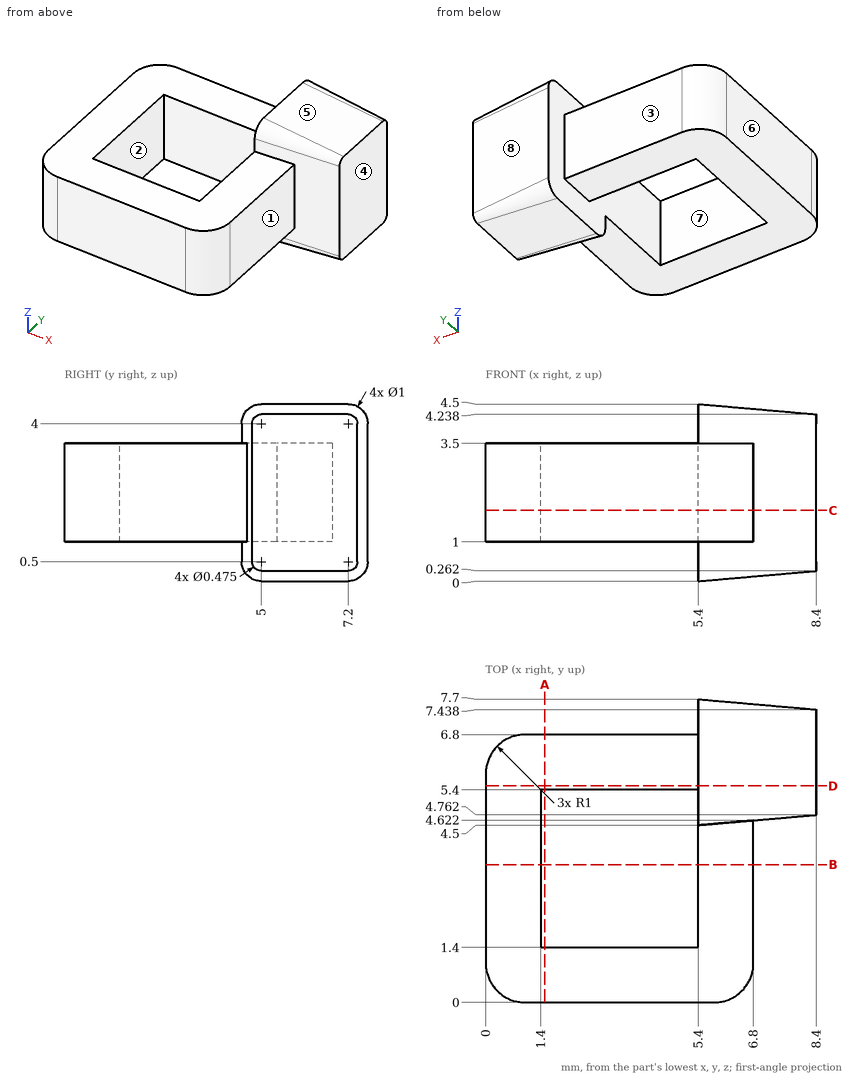
Could you check a few things on this drawing? It's one solid part, dimensions in mm from its lowest x, y, z. A direction names the side the tool comes from. Give positions to 0.01 mm unless a question says otherwise; leave off trailing zeros. Loops run counter-clockwise (first coordinate to the right, second up) from the corner with the lowest first, then second, coordinate; pieces in that order, holes last. Notation, with made-up numbers: M 75.25,-23.75 L 117.25,-23.75 A12 ccw 117.25,-9.75 Z; hole C 85.5,-14 d8. An arc over 180 degrees is marked long. Answer as a JSON object with one key per item and string values.
Q1. Suppose I cut it at D-D, the plane y = 5.5. List the corners of the cut face in (x, z) for me, plus the area to 3 significant figures.
Values found:
{"outline": "M 0,1 L 5.4,1 L 5.4,0 L 8.4,0.26 L 8.4,4.24 L 5.4,4.5 L 5.4,3.5 L 0,3.5 Z", "area": "26.2 mm²"}
Q2. Suppose I cut it at A-A, the plane x = 1.5. List the corners of the cut face in (y, z) for me.
Values found:
{"outline": "M 0,1 L 1.4,1 L 1.4,3.5 L 0,3.5 Z; M 5.4,1 L 6.8,1 L 6.8,3.5 L 5.4,3.5 Z"}
Q3. For the marked faces 1, 2, 3, 4 and 5, which set-ups out of +Z, -Z, +X, -X, +Y, -Y let a thin tool reach every point of the face, with its end or its side?
Values found:
{"face 1": "+Z, -Z, +X, -Y", "face 2": "+Z, -Z", "face 3": "+Z, -Z, -X, +Y", "face 4": "+Z, -Z, +X, +Y, -Y", "face 5": "+Z, +X, +Y, -Y"}
Q4. If I drill on probe 1 along X at (y, z) = (5.25, 1.8); probe 2 along Y at (x, z) = (3.25, 2), over which ranges is the centre line in solid material (lowest first)? Write a range as [from, to].
Values found:
{"probe 1": "x = [0, 1.4], [5.4, 8.4]", "probe 2": "y = [0, 1.4], [5.4, 6.8]"}
Q5. For P1, Ø2, axis at y = 2.5, z = 2.5, coming from the +X side; P2, Ø1, axis at x = 5, y = 3.5, coming from the +Z side; P3, Ø3, axis at x = 3, y = 3, coming from the +Z side; P4, Ø1.5, axis at x = 6.5, z = 0.5, coming from the +Y side, each with a flat end and sliding along its axis, tell me the tip position at first contact or that it passes through.
Values found:
{"P1": "stops at x = 6.8", "P2": "stops at z = 3.5", "P3": "passes through", "P4": "stops at y = 7.67"}
Q6. If we mould it in two halves opening along X, with no side actions, what happens to the marked faces 6, 7 and 8? For each: pulls with the +X half, pulls with the -X half, needs draft (parallel to the pull), parting line crosses it, or undercut.
Values found:
{"face 6": "pulls with the -X half", "face 7": "undercut", "face 8": "pulls with the +X half"}
Q7. Suppose I cut it at C-C, the plane z = 1.8. List the corners of the cut face in (x, y) for me.
Values found:
{"outline": "M 0,1 A1 ccw 1,0 L 5.8,0 A1 ccw 6.8,1 L 6.8,4.62 L 8.4,4.76 L 8.4,7.44 L 5.4,7.7 L 5.4,6.8 L 1,6.8 A1 ccw 0,5.8 Z; hole M 1.4,1.4 L 5.4,1.4 L 5.4,5.4 L 1.4,5.4 Z"}
